```python
from build123d import *

# Parameters (mm, degrees)
SKETCH2_R                = 13
SKETCH2_R_2              = 12.075
BOSS_EXTRUDE1_DEPTH      = 8
BOSS_EXTRUDE2_DEPTH      = 1
BOSS_EXTRUDE2_DEPTH_BACK = 1
SKETCH3_R                = 12.569499656
BOSS_EXTRUDE3_DEPTH      = 4
BOSS_EXTRUDE3_DEPTH_BACK = 4
SKETCH5_R                = 5.925
SKETCH5_R_2              = 5
SKETCH6_R                = 5
CUT_EXTRUDE1_DEPTH       = 2


with BuildPart() as part:
    # Sketch2 → Boss-Extrude1 (new body)
    with BuildSketch(Plane.XY):
        Circle(SKETCH2_R)
        Circle(SKETCH2_R_2, mode=Mode.SUBTRACT)
    extrude(amount=BOSS_EXTRUDE1_DEPTH)

    # Sketch3 → Boss-Extrude2 (add, two sides: drawn at the far end of the back side and taken through both)
    with BuildSketch(Plane(origin=(0, 0, 4), x_dir=(-1, 0, 0), z_dir=(0, 0, -1)).offset(-BOSS_EXTRUDE2_DEPTH_BACK)):
        Circle(SKETCH3_R)
    extrude(amount=BOSS_EXTRUDE2_DEPTH + BOSS_EXTRUDE2_DEPTH_BACK)

    # Sketch5 → Boss-Extrude3 (add, two sides: drawn at the far end of the back side and taken through both)
    with BuildSketch(Plane(origin=(0, 0, 4), x_dir=(-1, 0, 0), z_dir=(0, 0, -1)).offset(-BOSS_EXTRUDE3_DEPTH_BACK)):
        Circle(SKETCH5_R)
        Circle(SKETCH5_R_2, mode=Mode.SUBTRACT)
    extrude(amount=BOSS_EXTRUDE3_DEPTH + BOSS_EXTRUDE3_DEPTH_BACK)

    # Sketch6 → Cut-Extrude1 (cut)
    with BuildSketch(Plane.XY.offset(5)):
        with Locations(Location((0, 0, 0), (0, 0, 180))):
            Circle(SKETCH6_R)
    extrude(amount=-CUT_EXTRUDE1_DEPTH, mode=Mode.SUBTRACT)


solid = part.part
```
Model file for the job. Use its own axes, mm. A direction names the side the tool comes from. Round coordinates to 2 decimals unless told otherwise and drop trailing zeros. Loops run counter-clockwise (first coordinate to the right, second up) from the corner with the lowest first, then second, coordinate; pieces in that order, holes last. Notation, with made-up numbers: M 15.5,65 L 48.5,65 A21 ccw 48.5,80 Z; hole C -35.75,-5.75 d9. An arc over 180 degrees is marked long. Put each result on its own line as item: value. Start each with the question number.
Item 1: Drop flat-ended pins along their axis: P1, Ø4, axis at x = -5, z = 5, coming from the -Y side; P2, Ø1, axis at x = 6.5, z = 6, coming from the +Y side; P3, Ø1, axis at y = 3.5, z = 6, coming from the -X side. Give the stop position or say it passes through.
Item 2: Cut at A-A (x = 0). List the corners of the cut face in (y, z) (3 decimals).
Item 3: Mould opens along X. For faces 1 (the face through (-10.316, -7.91, 3.944)), 2 (the face through (-3, 6, 5)), 3 (the face through (9, -9, 0)) say: released by +X, released by -X, zero draft, split by the parting line, or undercut.
Item 4: Cut at D-D (y = -10). List the corners of the cut face in (x, z).
Item 5: 3-axis set-ups, long thin cutter, end or side, ignore diameter. For faces 4 (the face through (-5.65, 1.78, 1.52)), 5 (the face through (9, -9, 8)), 6 (the face through (-12.063, 0.531, 6.479)): which of +Z, -Z, +X, -X, +Y, -Y reach the whole face in a straight line?
Item 6: Drill centre lines: line 1 along Y through (x, z) = (0, 0.95) (3 decimals); line 2 along Y through (x, z) = (0, 4.5); line 3 along Y through (x, z) = (-1, 7). Where is each one in solid material? Low to high.
Item 7: Cut at C-C (z = 5.5). List the corners of the cut face in (x, y) (3 decimals).
Answer block:
1. P1: y = -12.65
1. P2: y = 11.53
1. P3: x = -12.65
2. outline: M -13,0 L -12.075,0 L -12.075,3 L -5.925,3 L -5.925,0 L -5,0 L -5,8 L -5.925,8 L -5.925,5 L -12.075,5 L -12.075,8 L -13,8 Z; M 5,0 L 5.925,0 L 5.925,3 L 12.075,3 L 12.075,0 L 13,0 L 13,8 L 12.075,8 L 12.075,5 L 5.925,5 L 5.925,8 L 5,8 Z
3. face 1: split by the parting line
3. face 2: undercut
3. face 3: zero draft
4. outline: M -8.31,0 L -6.77,0 L -6.77,3 L 6.77,3 L 6.77,0 L 8.31,0 L 8.31,8 L 6.77,8 L 6.77,5 L -6.77,5 L -6.77,8 L -8.31,8 Z
5. face 4: -Z
5. face 5: +Z, +X, -X, +Y, -Y
5. face 6: +Z
6. line 1: -13 to -12.075, -5.925 to -5, 5 to 5.925, 12.075 to 13
6. line 2: -13 to -5, 5 to 13
6. line 3: -12.96 to -12.03, -5.84 to -4.9, 4.9 to 5.84, 12.03 to 12.96
7. outline: C 0,0 d26; C 0,0 d11.85; hole C 0,0 d24.15; hole C 0,0 d10
